For this review, take the finished solid that the model builds, in its own axes (mm). A direction names the side the tool comes from. Coordinates: 2 decimals unless noted, no trailing zeros. Loops run counter-clockwise (first coordinate to the right, second up) from the corner with the lowest first, then second, coordinate; pieces in that order, holes last. Notation, with made-up numbers: M 16.5,-15 L 59.5,-15 A20 cw 59.5,8 Z; hole C -5,-4.5 d8. An arc over 180 degrees is marked long. Answer as a JSON object with one key per item and string values. Group by question number.
Item 1: Add section D-D (z = 0). Count the separate pieces of the cut face and the enclosed holes in it, then the cut area to 3 significant figures.
Item 2: Insertion check: pin 1 (8.5 mm diameter, centred on x = 40, z = -17, fed in from -Y); pin 2 (12 mm diameter, centred on y = 0.5, z = 2, fed in from -X); pin 3 (4 mm diameter, centred on x = 39.5, z = -14.5, fed in from +Y); pin 4 (2 mm diameter, centred on x = 23, y = 17, fed in from +Z). Each pin has a flat end and moves straight along its axis. Give the tip position at first contact, or say it passes through.
Item 3: Tool access review of faces 1 (the face through (34, 19, 0)), 2 (the face through (30.42, -10.469, 9.523)), 3 (the face through (44, -0.75, -16)), 4 (the face through (14.094, 19.138, 6.027)), 5 (the face through (59, 13, 0)): name each direction out of +Z, -Z, +X, -X, +Y, -Y from which nothing blocks a thin tool from reaching the whole face with its end or side.
Item 4: Add section C-C (x = 4.5). State the section outline as (y, z) points.
Item 5: Mouldability with a two-part tool opening along Y and no side actions: class faces 6 (the face through (4.93, -0.96, 34.31)), 7 (the face through (44.79, -19.48, -0.42)), 8 (the face through (12.028, 8.767, -16.856)) as +Y half, -Y half, draft (parallel to the pull), parting line (faces both ways), or undercut.
Item 6: Wall thickness on L1, parallel to X at y = 7, z = 27.5; L2, parallel to Y at x = 22, z = -1; L3, parallel to Y at x = 7.25, z = -32: over which ranges is each line inside the solid? List them lowest first. Write a range as from..to.
Item 7: Add section B-B (y = 30). State the section outline as (x, z) points, then the cut area to 3 significant figures.
Autodesk Inventor part; units mm, degrees
ref_plane "Work Plane1" through (0, 17.5, 0) normal (0, 1, 0) x (-1, 0, 0)
ref_plane "YZ Plane" through (0, 0, 0) normal (1, 0, 0) x (0, 1, 0)
ref_plane "XY Plane" through (0, 0, 0) normal (0, 0, 1) x (1, 0, 0)
sketch "Sketch1" plane through (0, 0, 0) normal (0, 0, 1) x (1, 0, 0)
  line L0 (0, 0) -> (60, 0)
  line L1 (0, 0) -> (0, 12.5) construction
  line L2 (0, 40) -> (10, 40)
  line L3 (10, 40) -> (10, 19)
  line L4 (10, 19) -> (14, 19)
  line L5 (0, 12.5) -> (60, 12.5)
  line L6 (60, 12.5) -> (60, 18.9524)
  line L7 (30, 20) -> (30, 19)
  line L8 (30, 19) -> (26, 19)
  line L9 (26, 19) -> (26, 19.9019)
  line L10 (14, 19.9019) -> (14, 19)
  line L11 (15.5, 22.5) -> (14, 19.9019)
  line L12 (15.5, 22.5) -> (24.5, 22.5)
  line L13 (24.5, 22.5) -> (26, 19.9019)
  line L14 (30, 20) -> (60, 18.9524)
  line L15 (30, 20) -> (60.0183, 20) construction
  arc A0 (0, 18.75) -> (0, 21.25) centre (0, 20) ccw
  line L16 (0, 12.5) -> (0, 18.75)
  line L17 (0, 21.25) -> (0, 40)
  dimension "d0" = 60
  dimension "d1" = 12.5
  dimension "d2" = 27.5
  dimension "d3" = 10
  dimension "d4" = 21
  dimension "d5" = 4
  dimension "d9" = 4
  dimension "d11" = 1
  dimension "d20" = 1.5
  dimension "d21" = 60
  dimension "d22" = 1.5
  dimension "d23" = 60
  dimension "d25" = 0.9019
  dimension "d26" = 0.9019
  dimension "d28" = 60
  dimension "d29" = 2
  dimension "d30" = 7.5
  dimension "d31" = 9
  dimension "d32" = 2.5
  dimension "d33" = 40
revolve "Revolution1" add sketch "Sketch1" angle 360 about axis through (0, 0, 0) along (1, 0, 0)
sketch "Sketch2" plane through (10, 0, 0) normal (1, 0, 0) x (0, 0, -1)
  point P0 (0, 0)
  point P1 (0, 32)
hole "Hole1" at (10, 32, 0) direction (-1, 0, 0) diameter 10.5 end through all
pattern_circular "Circular Pattern1" count 3 over 360 about axis through (30, 0, 0) along (1, 0, 0) of "Hole1"
sketch "Sketch3" plane through (10, 0, 0) normal (1, 0, 0) x (0, 0, -1)
  point P0 (0, 0)
  point P1 (0, 0)
  point P2 (32, 0)
hole "Hole2" at (10, 0, 0) at (10, 0, -32) direction (-1, 0, 0) diameter 5 end through all
pattern_circular "Circular Pattern2" count 2 over 360 about axis through (30, 0, 0) along (1, 0, 0) of "Hole2"
sketch "Sketch4" plane through (60, 0, 0) normal (1, 0, 0) x (0, 0, -1)
  line L0 (-62.0461, 0.75) -> (63.0717, 0.75)
  line L1 (63.0717, 0.75) -> (63.0717, -0.75)
  line L2 (63.0717, -0.75) -> (-62.0461, -0.75)
  line L3 (-62.0461, -0.75) -> (-62.0461, 0.75)
  point P0 (0, 0)
  dimension "d55" = 1.5
  dimension "d56" = 0.75
extrude "Extrusion1" cut sketch "Sketch4" against normal blind 32
sketch "Sketch5" plane through (60, 0, 0) normal (1, 0, 0) x (0, 0, -1)
  line L0 (0, 0) -> (-26.5, -45.8993)
  line L1 (0, 0) -> (53, 0) construction
  line L2 (-2.1416, -9.7648) -> (-5.1902, -14.9339)
  line L3 (-5.1902, -14.9339) -> (-10.3584, -11.8858)
  line L4 (-10.3584, -11.8858) -> (-7.3098, -6.7168)
  line L5 (-7.3098, -6.7168) -> (-2.1416, -9.7648)
  circle A0 centre (0, 0) radius 12.5
  line L6 (-2.1416, -9.7648) -> (-10.3584, -11.8858) construction
  line L7 (-5.1902, -14.9339) -> (-7.3098, -6.7168) construction
  point P0 (-6.25, -10.8253)
  dimension "d59" = 53
  dimension "d60" = 120
  dimension "d61" = 6
  dimension "d62" = 15.5
extrude "Extrusion2" cut sketch "Sketch5" against normal through all contours L5 L2 A0 L0 | L0 A0 L4 L5 | A0 L2 L3 L0 | L0 L3 L4 A0
chamfer "Chamfer1" distance 1.5 angle 45 3 edges at (60, -5.24, 11.3487) (60, 12.5, 0) (60, -10.2103, -7.2111)
thread "Thread1"
ref_plane "Work Plane1" through (0, 17.5, 0) normal (0, 1, 0) x (-1, 0, 0)
sketch "Sketch6" plane through (0, 17.5, 0) normal (0, 1, 0) x (-1, 0, 0)
  line L0 (-38, 0) -> (-50, 0) construction
  line L1 (-38, 4) -> (-50, 4)
  line L2 (-50, -4) -> (-38, -4)
  arc A0 (-38, -4) -> (-38, 4) centre (-38, 0) ccw
  arc A1 (-50, 4) -> (-50, -4) centre (-50, 0) ccw
  point P0 (0, 0)
  point P1 (-44, 0)
  dimension "d71" = 8
  dimension "d72" = 38
  dimension "d73" = 50
extrude "Extrusion3" cut sketch "Sketch6" along normal blind 26.5
equation "\"d22\" = d20"
equation "\"d23\" = d21"
equation "\"d26\" = d25"
properties part number "Spannhylsa_2015_HT1"
From the geometry:
{
 "1": {"separate pieces": "3", "enclosed holes": "0", "area": "1,150 mm²"},
 "2": {"pin 1": "stops at y = -14.96", "pin 2": "passes through", "pin 3": "stops at y = 15.19", "pin 4": "stops at z = 15.82"},
 "3": {"face 1": "+Y", "face 2": "+X, -X", "face 3": "+Z, -Z, +X", "face 4": "none", "face 5": "+X"},
 "4": {"outline": "C 0,0 d80; hole C -16,-27.71 d10.5; hole C -16,27.71 d10.5; hole M -14.93,5.19 L -12.01,3.47 A12.5 ccw long -9.01,8.66 L -11.89,10.36 Z; hole C 0,-32 d5; hole C 0,32 d5; hole C 32,0 d10.5"},
 "5": {"face 6": "undercut", "face 7": "-Y half", "face 8": "parting line"},
 "6": {"L1": "x = 0..10", "L2": "y = -22.48..-12.46, 12.46..22.48", "L3": "y = -24..-19.03, -12.97..-2.5, 2.5..24"},
 "7": {"outline": "M 0,-26.46 L 10,-26.46 L 10,-4.85 L 0,-4.85 Z; M 0,4.85 L 10,4.85 L 10,26.46 L 0,26.46 Z", "area": "432 mm²"}
}
